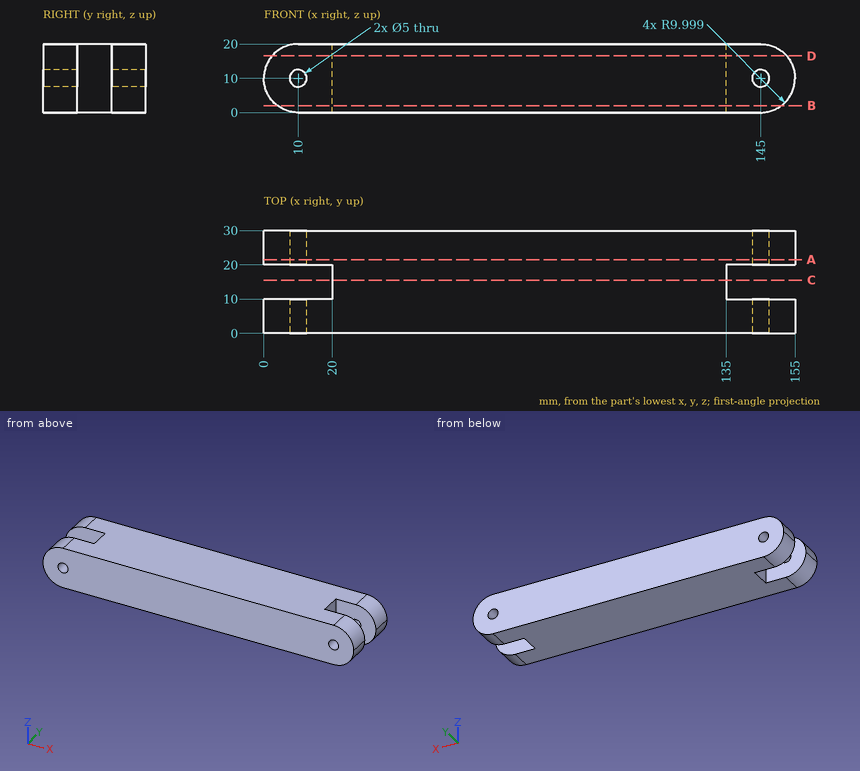
Print and shaded views of the part. All mm, measured from the part's lowest x, y and z. Give positions to 0.01 mm unless a question says otherwise; leave off trailing zeros. Order: outer loops, then holes, each group sorted by start corner. A loop starts at its lowest first (then second) coordinate and runs counter-clockwise, first axis right, second up. Notation, with made-up numbers: (1, 35) - (36, 35) arc R36 cw to (36, 73) - close; hole circle Ø6 at (43, -2). An arc over 180 degrees is marked (long way). Use a Markdown table: item, result.
1) Saw through at B-B on z = 2. List the corners of the cut face in (x, y), plus the area to 3 significant figures.
Checked values:
| item | result |
|---|---|
| outline | (4, 0) - (151, 0) - (151, 10) - (135, 10) - (135, 20) - (151, 20) - (151, 30) - (4, 30) - (4, 20) - (20, 20) - (20, 10) - (4, 10) - close |
| area | 4,090 mm² |
2) Flat gauge pins, fed straight in: P1, Ø3, axis at x = 10, z = 10, coming from the -Y side; P2, Ø2, axis at y = 14, z = 5.5, coming from the +X side; P3, Ø5, axis at y = 7.5, z = 13, coming from the -X side; P4, Ø12, axis at y = 8, z = 3, coming from the -X side. Where does each tip first touch, or does it go through?
Checked values:
| item | result |
|---|---|
| P1 | through |
| P2 | x = 135 |
| P3 | x = 0.01 |
| P4 | x = 0.05 |
3) Saw through at A-A on y = 21.5. Count the separate pieces of the cut face and the enclosed holes in it, plus the area to 3 significant figures.
Checked values:
| item | result |
|---|---|
| separate pieces | 1 |
| enclosed holes | 2 |
| area | 2,970 mm² |
4) Probe L1, parallel to Y at x = 9.5, z = 7.5; L2, parallel to Z at x = 10, y = 2; L3, parallel to X at y = 13.25, z = 17. List the from-to ranges inside material, lowest first. Write a range as from..to.
Checked values:
| item | result |
|---|---|
| L1 | 0..10, 20..30 |
| L2 | 0..7.5, 12.5..20 |
| L3 | 20..135 |
5) Saw through at D-D on z = 16.5. List the corners of the cut face in (x, y).
Checked values:
| item | result |
|---|---|
| outline | (2.4, 0) - (152.6, 0) - (152.6, 10) - (135, 10) - (135, 20) - (152.6, 20) - (152.6, 30) - (2.4, 30) - (2.4, 20) - (20, 20) - (20, 10) - (2.4, 10) - close |
6) Saw through at C-C on y = 15.5. List the corners of the cut face in (x, z), plus the area to 3 significant figures.
Checked values:
| item | result |
|---|---|
| outline | (20, 0) - (135, 0) - (135, 20) - (20, 20) - close |
| area | 2,300 mm² |
